Geometry check sheet. Reference: the model listing, model coordinates, mm. Face numbers are marked on the shaded views. A direction names the side the tool comes from. Round coordinates to 2 decimals unless told otherwise and drop trailing zeros. Write each loop counter-clockwise with the first axis right and the second up, starting at its lowest first coordinate (ties: lowest second). Pieces come first, ordered by that corner, then holes. Notation, with made-up numbers: M 12,85 L 64,85 A10 ccw 64,98 Z; hole C 76.25,81.5 d9. An arc over 180 degrees is marked long. Use a Markdown table: item, result.
```python
from build123d import *

# Parameters (mm, degrees)
F1_DEPTH  = 1.6
F3_DEPTH  = 10.5
F5_START  = 35
F5_DEPTH  = 6.5
F6_W      = 3.2
F6_H      = 3.5
F7_DEPTH  = 3.6
F8_W      = 3
F8_H      = 4.3
F9_DEPTH  = 4.5
F10_W     = 5.15
F10_H     = 6.15
F10_W_2   = 6.15
F10_H_2   = 5.15
F11_DEPTH = 1.1


with BuildPart() as f1:
    # F0 (on Top) → F1 (new body)
    with BuildSketch(Plane.XY):
        with BuildLine():
            Line((1.2, 15.2), (0.7727922061, 15.2))
            ThreePointArc((0.7727922061, 15.2), (0.4943088368, 15.2847326006), (0.3102119479, 15.5102119479))
            Line((0.3102119479, 15.5102119479), (-0.3102119479, 14.8897880521))
            ThreePointArc((-0.3102119479, 14.8897880521), (-0.0847326006, 14.7056911632), (0, 14.4272077939))
            Line((0, 14.4272077939), (0, 4.05))
            Line((0, 4.05), (5.2, 4.05))
            ThreePointArc((5.2, 4.05), (5.5535533906, 3.9035533906), (5.7, 3.55))
            Line((5.7, 3.55), (5.7, 3.35))
            ThreePointArc((5.7, 3.35), (5.5535533906, 2.9964466094), (5.2, 2.85))
            Line((5.2, 2.85), (1.7, 2.85))
            ThreePointArc((1.7, 2.85), (1.5535533906, 2.4964466094), (1.2, 2.35))
            Line((1.2, 2.35), (0, 2.35))
            Line((0, 2.35), (0, 0.7727922061))
            ThreePointArc((0, 0.7727922061), (-0.0847326006, 0.4943088368), (-0.3102119479, 0.3102119479))
            Line((-0.3102119479, 0.3102119479), (0.3102119479, -0.3102119479))
            ThreePointArc((0.3102119479, -0.3102119479), (0.4943088368, -0.0847326006), (0.7727922061, 0))
            Line((0.7727922061, 0), (1.2, 0))
            Line((1.2, 0), (33.8, 0))
            Line((33.8, 0), (34.2272077939, 0))
            ThreePointArc((34.2272077939, 0), (34.5056911632, -0.0847326006), (34.6897880521, -0.3102119479))
            Line((34.6897880521, -0.3102119479), (35.3102119479, 0.3102119479))
            ThreePointArc((35.3102119479, 0.3102119479), (35.0847326006, 0.4943088368), (35, 0.7727922061))
            Line((35, 0.7727922061), (35, 3.85))
            Line((35, 3.85), (30, 3.85))
            ThreePointArc((30, 3.85), (29.6464466094, 3.9964466094), (29.5, 4.35))
            Line((29.5, 4.35), (29.5, 4.55))
            ThreePointArc((29.5, 4.55), (29.6464466094, 4.9035533906), (30, 5.05))
            Line((30, 5.05), (35, 5.05))
            Line((35, 5.05), (35, 14.4272077939))
            ThreePointArc((35, 14.4272077939), (35.0847326006, 14.7056911632), (35.3102119479, 14.8897880521))
            Line((35.3102119479, 14.8897880521), (34.6897880521, 15.5102119479))
            ThreePointArc((34.6897880521, 15.5102119479), (34.5056911632, 15.2847326006), (34.2272077939, 15.2))
            Line((34.2272077939, 15.2), (33.8, 15.2))
            Line((33.8, 15.2), (1.2, 15.2))
        make_face()
    extrude(amount=F1_DEPTH)

    # F2 (on Right) → F3 (join)
    with BuildSketch(Plane.YZ):
        Polygon((7.35, 4), (0.85, 4), (0.85, -3.7), (7.35, -3.7), (7.35, -3.1), (14.35, -3.1), (14.35, 3.4), (7.35, 3.4), align=None)
    extrude(amount=-F3_DEPTH)

    # F4 (on Right) → F5 (join)
    with BuildSketch(Plane.YZ.offset(F5_START)):
        Polygon((7.55, 2.95), (0.85, 2.95), (0.85, -4.65), (7.55, -4.65), (7.55, -4), (14.35, -4), (14.35, 2.3), (7.55, 2.3), align=None)
    extrude(amount=F5_DEPTH)

    # F6 (on Top) → F7 (join)
    with BuildSketch(Plane.XY):
        with Locations((32.15, 1.8)):
            Rectangle(F6_W, F6_H)
        with BuildLine():
            ThreePointArc((30.9, 2.5), (31.1050252532, 2.9949747468), (31.6, 3.2))
            Line((31.6, 3.2), (32.7, 3.2))
            ThreePointArc((32.7, 3.2), (33.1949747468, 2.9949747468), (33.4, 2.5))
            Line((33.4, 2.5), (33.4, 1.1))
            ThreePointArc((33.4, 1.1), (33.1949747468, 0.6050252532), (32.7, 0.4))
            Line((32.7, 0.4), (31.6, 0.4))
            ThreePointArc((31.6, 0.4), (31.1050252532, 0.6050252532), (30.9, 1.1))
            Line((30.9, 1.1), (30.9, 2.5))
        make_face(mode=Mode.SUBTRACT)
    extrude(amount=F7_DEPTH)

    # F8 (on Top) → F9 (join)
    with BuildSketch(Plane.XY):
        with Locations((25.5, 12.95)):
            Rectangle(F8_W, F8_H)
    extrude(amount=-F9_DEPTH)

    # F10 (on Top) → F11 (join)
    with BuildSketch(Plane.XY):
        with Locations((10.9508251641, 9.2315472887)):
            Rectangle(F10_W, F10_H)
        with Locations((16.9374256049, 10.8333893863)):
            Rectangle(F10_W, F10_H)
        with Locations((17.7855274571, 3.0699999196)):
            Rectangle(F10_W_2, F10_H_2)
    extrude(amount=-F11_DEPTH)


solid = f1.part
```
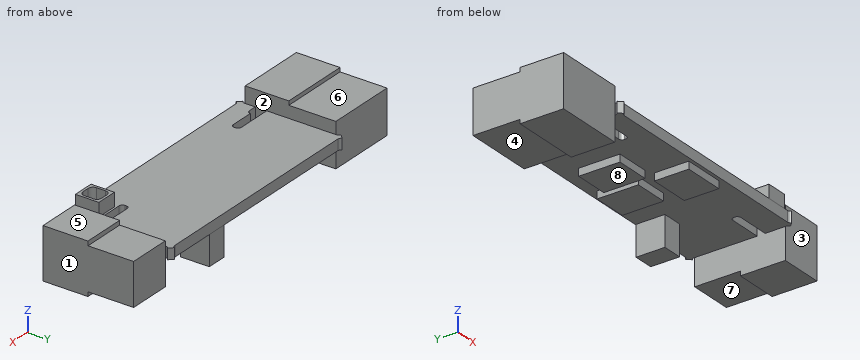
Item 1: Cross-section at D-D, the plane x = 22. Record the cut outline in (y, z).
Outcome:
| item | result |
|---|---|
| outline | M 0,0 L 15.2,0 L 15.2,1.6 L 0,1.6 Z |
Item 2: Go/stop test with flat-tipped pins: pin 1 (7 mm diameter, centred on x = 38.5, y = 11.5, fed in from +Z); pin 2 (2 mm diameter, centred on x = 40, z = -1, fed in from -Y); pin 3 (5 mm diameter, centred on x = -3, z = 1, fed in from +Y). Record where each tip stops, or that it passes through.
Outcome:
| item | result |
|---|---|
| pin 1 | stops at z = 2.3 |
| pin 2 | stops at y = 0.85 |
| pin 3 | stops at y = 14.35 |
Item 3: Mould release check, pull along X, two halves, no side actions. Record for the marked faces 1, 2 and 3: +X half, -X half, draft (parallel to the pull), parting line (faces both ways), or undercut.
Outcome:
| item | result |
|---|---|
| face 1 | +X half |
| face 2 | undercut |
| face 3 | draft |
Item 4: Access from +Z, -Z, +X, -X, +Y, -Y to the whole of each face (thin tool, end or side, straight path). Record for the marked faces 4, 5, 6, 7 and 8.
Outcome:
| item | result |
|---|---|
| face 4 | -Z, -X, +Y |
| face 5 | +Z, +X, +Y, -Y |
| face 6 | +Z, +X, -X, +Y |
| face 7 | -Z, +X, +Y |
| face 8 | -Z, +Y, -Y |
Item 5: Cross-section at C-C, the plane y = 10. Record the cut outline in (x, z), and give its area (3 significant figures).
Outcome:
| item | result |
|---|---|
| outline | M -10.5,-3.1 L 0,-3.1 L 0,0 L 8.38,0 L 8.38,-1.1 L 13.53,-1.1 L 13.53,0 L 14.36,0 L 14.36,-1.1 L 19.51,-1.1 L 19.51,0 L 35,0 L 35,-4 L 41.5,-4 L 41.5,2.3 L 35,2.3 L 35,1.6 L 0,1.6 L 0,3.4 L -10.5,3.4 Z |
| area | 177 mm2 |
Item 6: Cross-section at A-A, the plane z = -1.75. Record the cut outline in (x, y), and give its area (3 significant figures).
Outcome:
| item | result |
|---|---|
| outline | M -10.5,0.85 L 0,0.85 L 0,14.35 L -10.5,14.35 Z; M 24,10.8 L 27,10.8 L 27,15.1 L 24,15.1 Z; M 35,0.85 L 41.5,0.85 L 41.5,14.35 L 35,14.35 Z |
| area | 242 mm2 |
Item 7: Material ranges on line 1 along X through (y, z) = (12.5, -2.25); line 2 along X through (y, z) = (2.75, -0.5); line 3 along X through (y, z) = (7.75, 2.25), recorded low to high. Write a range as from..to.
Outcome:
| item | result |
|---|---|
| line 1 | x = -10.5..0, 24..27, 35..41.5 |
| line 2 | x = -10.5..0, 14.71..20.86, 35..41.5 |
| line 3 | x = -10.5..0, 35..41.5 |
Item 8: Cross-section at B-B, the plane x = 38.5. Record the cut outline in (y, z).
Outcome:
| item | result |
|---|---|
| outline | M 0.85,-4.65 L 7.55,-4.65 L 7.55,-4 L 14.35,-4 L 14.35,2.3 L 7.55,2.3 L 7.55,2.95 L 0.85,2.95 Z |
